Check sheet for the modelled part. Datum: model origin and axes. Units: mm. Face numbers are marked on the shaded views. A direction names the side the tool comes from. Round coordinates to 2 decimals unless told otherwise and drop trailing zeros. Order: outer loops, then holes, each group sorted by start corner. A loop starts at its lowest first (then second) coordinate and runs counter-clockwise, first axis right, second up.
Q1. Cross-section at D-D on z = 25. Record the cut outline in (x, y).
Q2. Scan lines: probe 1 along Z at (x, y) = (9.5, -6); probe 2 along X at (y, z) = (-9, 1); probe 3 along Y at (x, z) = (30, 5). Record each from-to range of solid material in increasing order.
Q3. Depth check by flat-ended pin: P1, Ø3, axis at x = 12, y = -12, coming from the +Z side; P2, Ø4, axis at x = 27, z = -2, coming from the -Y side; P3, Ø4, axis at x = 6.5, z = -8, coming from the +Y side; P4, Ø2, axis at y = 9, z = 2.5, coming from the -X side. Enter the tip coordinate at first touch or a pass-through.
Q4. Cross-section at A-A on z = -1.5. Record the cut outline in (x, y).
Q5. Mould release check, pull along X, two halves, no side actions. Record for the marked faces 1, 2 and 3: +X half, -X half, draft (parallel to the pull), parting line (faces both ways), or undercut.
Q6. Set-up check for the marked faces 4, 5 and 6: record each of +Z, -Z, +X, -X, +Y, -Y from which the full face is reachable in a straight line by a thin tool's end or side.
Q7. Cross-section at B-B on x = 0. Record the cut outline in (y, z).
Q8. Cross-section at C-C on y = -4.5. Record the cut outline in (x, z).
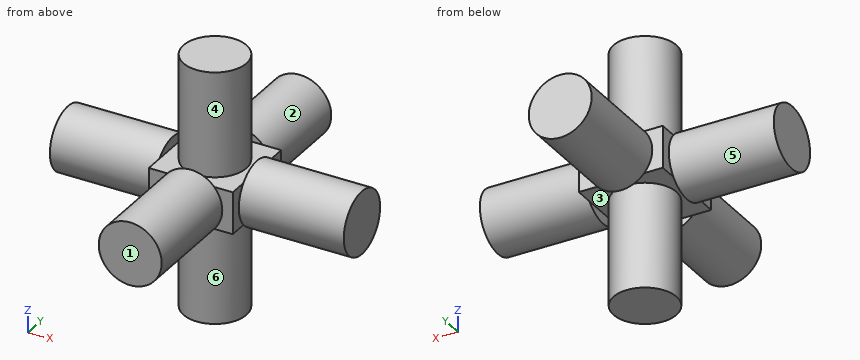
from build123d import *

# Parameters (mm, degrees)
F0_W      = 20
F0_H      = 20
F1_DEPTH  = 10
F2_R      = 7.5
F8_DEPTH  = 25
F3_R      = 7.5
F9_DEPTH  = 25
F4_R      = 7.5
F10_DEPTH = 25
F5_R      = 7.5
F11_DEPTH = 25
F6_R      = 7.5
F12_DEPTH = 25
F7_R      = 7.5
F13_DEPTH = 25


with BuildPart() as f1:
    # F0 (on Top) → F1 (new body)
    with BuildSketch(Plane.XY):
        Rectangle(F0_W, F0_H)
    extrude(amount=F1_DEPTH)

    # F2 (on face) → F8 (join)
    with BuildSketch(Plane.XY.offset(10)):
        Circle(F2_R)
    extrude(amount=F8_DEPTH)

    # F3 (on face) → F9 (join)
    with BuildSketch(Plane(origin=(0, 10, 0), x_dir=(-1, 0, 0), z_dir=(0, 1, 0))):
        with Locations((0, 5)):
            Circle(F3_R)
    extrude(amount=F9_DEPTH)

    # F4 (on face) → F10 (join)
    with BuildSketch(Plane.XZ.offset(10)):
        with Locations((0, 5)):
            Circle(F4_R)
    extrude(amount=F10_DEPTH)

    # F5 (on face) → F11 (join)
    with BuildSketch(Plane(origin=(-10, 0, 0), x_dir=(0, -1, 0), z_dir=(-1, 0, 0))):
        with Locations((0, 5)):
            Circle(F5_R)
    extrude(amount=F11_DEPTH)

    # F6 (on face) → F12 (join)
    with BuildSketch(Plane.YZ.offset(10)):
        with Locations((0, 5)):
            Circle(F6_R)
    extrude(amount=F12_DEPTH)

    # F7 (on face) → F13 (join)
    with BuildSketch(Plane.XY):
        Circle(F7_R)
    extrude(amount=-F13_DEPTH)


solid = f1.part
Results found:
1. outline: circle Ø15 at (0, 0)
2. probe 1: z = 0 to 10
2. probe 2: x = -10 to 10
2. probe 3: y = -7.5 to 7.5
3. P1: passes through
3. P2: stops at y = -5.59
3. P3: stops at y = 6
3. P4: stops at x = -10
4. outline: (-35, -3.74) - (-10, -3.74) - (-10, 3.74) - (-35, 3.74) - close; circle Ø15 at (0, 0); (-3.74, -35) - (3.74, -35) - (3.74, -10) - (-3.74, -10) - close; (-3.74, 10) - (3.74, 10) - (3.74, 35) - (-3.74, 35) - close; (10, -3.74) - (35, -3.74) - (35, 3.74) - (10, 3.74) - close
5. face 1: draft
5. face 2: parting line
5. face 3: undercut
6. face 4: +Z
6. face 5: -X
6. face 6: -Z
7. outline: (-35, -2.5) - (-10, -2.5) - (-10, 0) - (-7.5, 0) - (-7.5, -25) - (7.5, -25) - (7.5, 0) - (10, 0) - (10, -2.5) - (35, -2.5) - (35, 12.5) - (10, 12.5) - (10, 10) - (7.5, 10) - (7.5, 35) - (-7.5, 35) - (-7.5, 10) - (-10, 10) - (-10, 12.5) - (-35, 12.5) - close
8. outline: (-35, -1) - (-10, -1) - (-10, 0) - (-6, 0) - (-6, -25) - (6, -25) - (6, 0) - (10, 0) - (10, -1) - (35, -1) - (35, 11) - (10, 11) - (10, 10) - (6, 10) - (6, 35) - (-6, 35) - (-6, 10) - (-10, 10) - (-10, 11) - (-35, 11) - close
